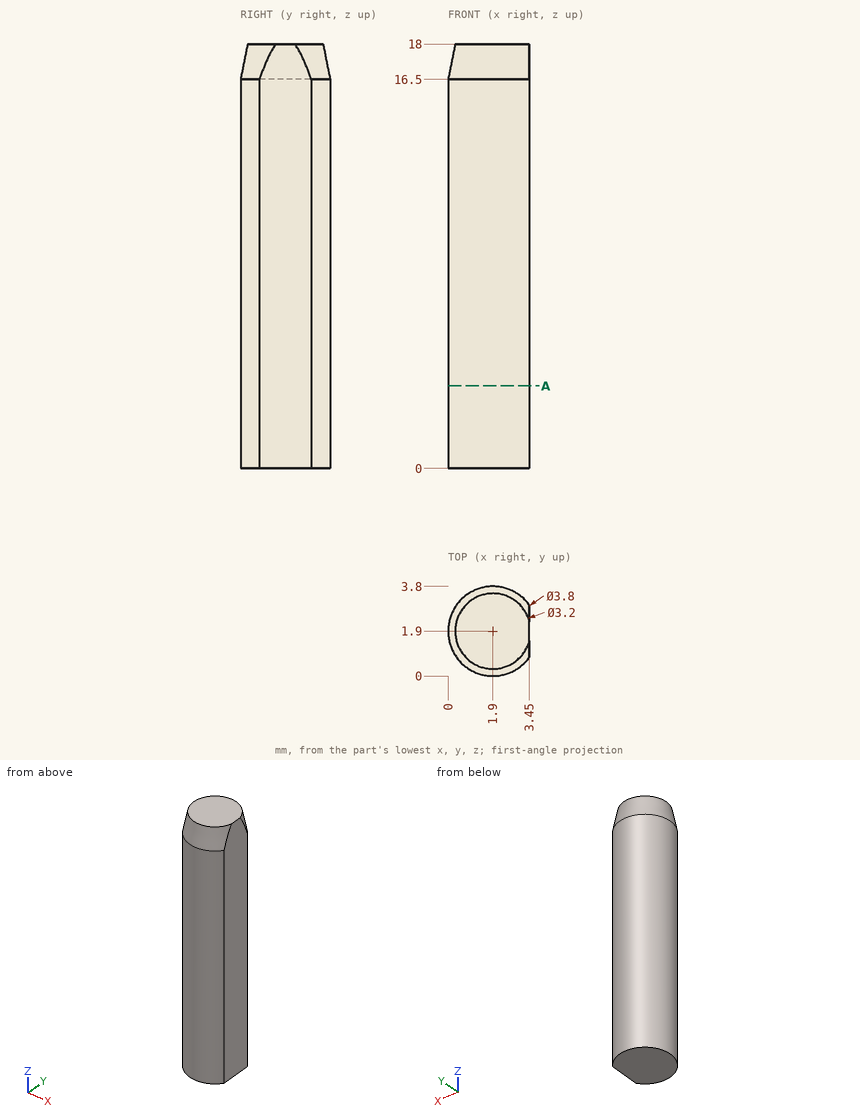
Check sheet for the drawn part. Datum: minimum x, y, z corner. Units: mm. Give positions to 0.01 mm unless a question says otherwise; leave off trailing zeros. Loops run counter-clockwise (first coordinate to the right, second up) from the corner with the lowest first, then second, coordinate; pieces in that order, holes last. Notation, with made-up numbers: M -21.5,44.25 L 8.5,44.25 A4 ccw 8.5,50.25 Z; hole C 68.5,33 d5. An arc over 180 degrees is marked long. Return JSON: item names as keys, results as strings.
1) Gauge pin test, flat end, axial feed: P1, Ø1.5, axis at x = 2.5, y = 1, coming from the -Z side. Record the tip position at first contact, or that the pin passes through.
Findings:
{"P1": "stops at z = 0"}
2) Material ranges on L1, parallel to X at y = 1.8, z = 10.75; L2, parallel to X at y = 1.4, z = 7.75; L3, parallel to Y at x = 2.4, z = 1.25, recorded low to high. Write a range as [from, to].
Findings:
{"L1": "x = [0, 3.45]", "L2": "x = [0.07, 3.45]", "L3": "y = [0.07, 3.73]"}
3) Section check A-A, the plane z = 3.5. Enter the section's corners in (x, y).
Findings:
{"outline": "M 3.45,0.8 L 3.45,3 A1.9 ccw long Z"}
